The listing builds one solid part. Answer for the finished solid, in the listing's coordinates (mm). Face numbers are marked on the shaded views. A direction names the side the tool comes from. Give positions to 0.01 mm unless a question says otherwise; leave off trailing zeros. Order: outer loops, then holes, each group sorted by start corner. A loop starts at its lowest first (then second) coordinate and runs counter-clockwise, first axis right, second up. Notation, with made-up numbers: (52.25, 75.5) - (100.25, 75.5) arc R35 ccw to (100.25, 114.5) - close; hole circle Ø4 at (35.5, 10.25). An arc over 180 degrees is marked (long way). Answer as CSV lines item,"result". Start each with the question number.
1. Section C-C on y = 0 is taken. Give the vertices of the cut face in (x, z) (3 decimals), and give its area (3 significant figures).
2. Section A-A on x = -15.5 is taken. Give the vertices of the cut face in (y, z), and give its area (3 significant figures).
3. Flat-ended cylindrical pins translate along their axes: pin 1 (12 mm diameter, centred on y = -3, z = -28, fed in from -X); pin 2 (6.5 mm diameter, centred on x = 28, y = -3.5, fed in from -Z); pin 3 (4.5 mm diameter, centred on x = 15.5, z = -6.15, fed in from +Y). Find the tip coordinate at first contact, or state that the pin passes through.
4. Which of the six approach directions +Z, -Z, +X, -X, +Y, -Y give full straight-line access (tool end or side, diameter ignored) to the marked faces 5, 6 and 7?
5. Consider line 1 along Z through (x, y) = (15.5, -18.85); line 2 along X through (y, z) = (1.5, -8); line 3 along Z through (x, y) = (-15, -19). Determine where each line is inside the solid, lowest interval first. Write a range as [from, to].
6. Determine the mould class of the marked faces 1, 2, 3 and 4 for opening direction X: +X half, -X half, draft (parallel to the pull), parting line (faces both ways), or undercut.
7. Section D-D on z = -10 is taken. Give the vertices of the cut face in (x, y).
8. Section B-B on x = 0 is taken. Give the vertices of the cut face in (y, z), and give its area (3 significant figures).
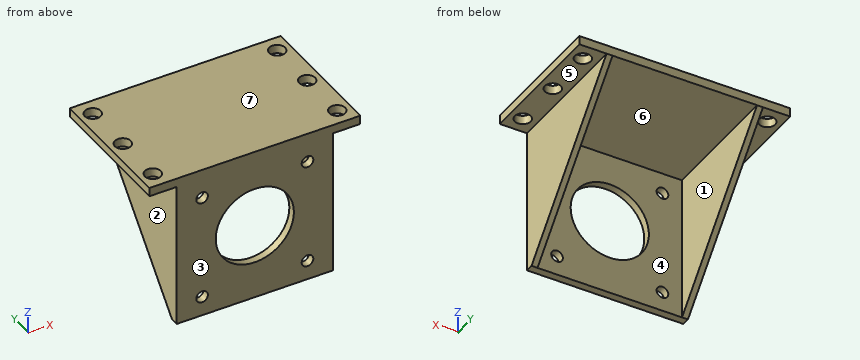
from build123d import *

# Parameters (mm, degrees)
SKETCH_W             = 62
SKETCH_H             = 40
PAD_DEPTH            = 2.59
PAD001_DEPTH         = 23
SKETCH003_R          = 2.3495
HOLE_DEPTH           = 175.977346
SKETCH004_R          = 1.7145
HOLE001_DEPTH        = 20.001
SKETCH005_R          = 11.5
POCKET_DEPTH         = 20.001
SKETCH006_W          = 42.5
SKETCH006_H          = 100
POCKET001_DEPTH      = 100
POCKET001_DEPTH_BACK = -17.714


with BuildPart() as part:
    # Sketch → Pad (new body)
    with BuildSketch(Plane.XY):
        Rectangle(SKETCH_W, SKETCH_H)
    extrude(amount=PAD_DEPTH)

    # Sketch001 → Pad001 (join, symmetric)
    with BuildSketch(Plane.YZ):
        Polygon((-20, -42.926), (-17.714, -42.926), (20, 0), (-20, 2.59), align=None)
    extrude(amount=PAD001_DEPTH, both=True)

    # Sketch003 → Hole (cut, through all)
    with BuildSketch(Plane.XY):
        with Locations((27.1145, 15.1003)):
            Circle(SKETCH003_R)
        with Locations((27.1145, -15.1003)):
            Circle(SKETCH003_R)
        with Locations((27.1145, 0)):
            Circle(SKETCH003_R)
    hole = extrude(amount=HOLE_DEPTH, mode=Mode.SUBTRACT)

    # Mirrored001: Hole across YZ
    add(hole.mirror(Plane.YZ), mode=Mode.SUBTRACT)

    # Sketch004 → Hole001 (cut, through all)
    with BuildSketch(Plane.XZ):
        with Locations((-15.5, -6.1468)):
            Circle(SKETCH004_R)
        with Locations((-15.5, -37.1468)):
            Circle(SKETCH004_R)
        with Locations((15.5, -37.1468)):
            Circle(SKETCH004_R)
        with Locations((15.5, -6.1468)):
            Circle(SKETCH004_R)
    extrude(amount=HOLE001_DEPTH, mode=Mode.SUBTRACT)

    # Sketch005 → Pocket (cut, through all)
    with BuildSketch(Plane.XZ):
        with Locations((0, -20.5)):
            Circle(SKETCH005_R)
    extrude(amount=POCKET_DEPTH, mode=Mode.SUBTRACT)

    # Sketch006 → Pocket001 (cut, two sides)
    with BuildSketch(Plane.XZ) as pocket001_sk:
        with Locations((0, -50)):
            Rectangle(SKETCH006_W, SKETCH006_H)
    extrude(amount=-POCKET001_DEPTH, mode=Mode.SUBTRACT)
    extrude(pocket001_sk.sketch, amount=-POCKET001_DEPTH_BACK, mode=Mode.SUBTRACT)


solid = part.part
Checks:
1,outline,"(-31, 0) - (-29.464, 0) - (-29.464, 2.59) - (-31, 2.59) - close; (-24.765, 0) - (-23, 0) - (-23, -22.764) - (-21.25, -22.764) - (-21.25, 0) - (21.25, 0) - (21.25, -22.764) - (23, -22.764) - (23, 0) - (24.765, 0) - (24.765, 2.59) - (-24.765, 2.59) - close; (29.464, 0) - (31, 0) - (31, 2.59) - (29.464, 2.59) - close"
1,area,"216 mm²"
2,outline,"(-20, -42.93) - (-17.71, -42.93) - (-17.71, -38.86) - (-20, -38.86) - close; (-20, -35.43) - (-17.71, -35.43) - (-17.71, -7.86) - (-20, -7.86) - close; (-20, -4.43) - (-17.71, -4.43) - (-17.71, 0) - (20, 0) - (20, 2.59) - (-20, 2.59) - close"
2,area,"186 mm²"
3,pin 1,"stops at x = -23"
3,pin 2,"stops at z = 0"
3,pin 3,"stops at y = -17.71"
4,face 5,"-Z, +X, +Y, -Y"
4,face 6,"-Z, +Y"
4,face 7,"+Z, +X, -X, +Y, -Y"
5,line 1,"z = [-42.93, -38.86], [-35.43, -7.86], [-4.43, 2.59]"
5,line 2,"x = [-23, -21.25], [21.25, 23]"
5,line 3,"z = [-42.93, -38.79], [-35.51, -7.79], [-4.51, 2.59]"
6,face 1,"undercut"
6,face 2,"-X half"
6,face 3,"draft"
6,face 4,"undercut"
7,outline,"(-23, -20) - (-4.69, -20) - (-4.69, -17.71) - (-21.25, -17.71) - (-21.25, 11.21) - (-23, 11.21) - close; (4.69, -20) - (23, -20) - (23, 11.21) - (21.25, 11.21) - (21.25, -17.71) - (4.69, -17.71) - close"
8,outline,"(-20, -42.93) - (-17.71, -42.93) - (-17.71, -32) - (-20, -32) - close; (-20, -9) - (-17.71, -9) - (-17.71, 0) - (20, 0) - (20, 2.59) - (-20, 2.59) - close"
8,area,"149 mm²"
